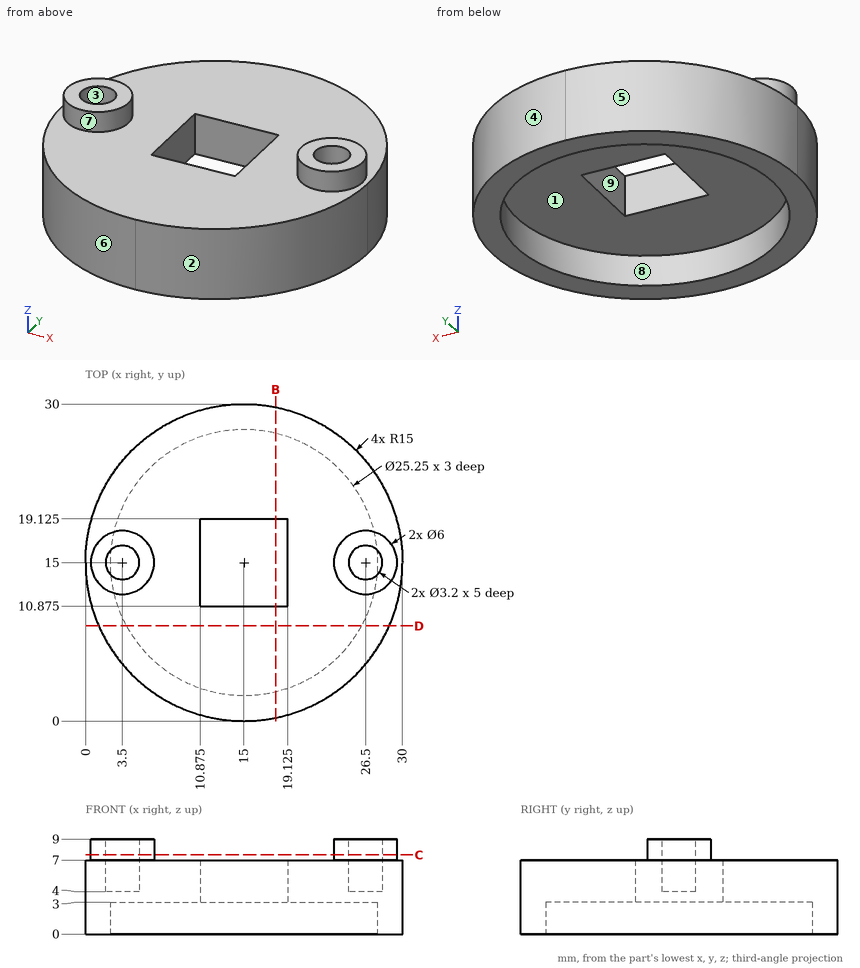
Can you work these out from the drawing? Everything is in mm from the part's minimum corner. A direction names the side the tool comes from. Give positions to 0.01 mm unless a question says otherwise; leave off trailing zeros. Loops run counter-clockwise (first coordinate to the right, second up) from the corner with the lowest first, then second, coordinate; pieces in that order, holes last. Notation, with made-up numbers: (4.25, 77) -> (61.25, 77) arc R7 ccw to (61.25, 82) -> close; hole circle Ø8 at (-27.75, 37.25). An arc over 180 degrees is marked (long way). Write item = value, one per line.
1) Will these pins go through, and if not, where does the flat tip stop? pin 1 (1.5 mm diameter, centred on x = 26, z = 2.5, fed in from -Y); pin 2 (3 mm diameter, centred on x = 3.5, y = 15, fed in from +Z); pin 3 (5 mm diameter, centred on x = 7, y = 8.5, fed in from +Z); pin 4 (5 mm diameter, centred on x = 14, z = 8, fed in from -Y).
Check result:
pin_1 = 4.05
pin_2 = 4
pin_3 = 7
pin_4 = 0
2) For the marked faces 5, 6, 7, 8 and 9, which set-ups out of +Z, -Z, +X, -X, +Y, -Y let a thin tool reach every point of the face, with its end or its side?
Check result:
face_5 = +Z, -Z, -X, +Y
face_6 = +Z, -Z, -X, -Y
face_7 = +Z
face_8 = -Z
face_9 = +Z, -Z
3) Suppose I cut it at C-C on z = 7.5. Write out the boundary of the cut face in (x, y).
Check result:
outline = circle Ø6 at (3.5, 15); circle Ø6 at (26.5, 15); hole circle Ø3.2 at (3.5, 15); hole circle Ø3.2 at (26.5, 15)
4) Thinking about a two-plate mould opening in Y: for the marked faces 1, 2, 3 and 4, which applies, released by +Y, released by -Y, zero draft, split by the parting line, or undercut?
Check result:
face_1 = undercut
face_2 = released by -Y
face_3 = undercut
face_4 = released by +Y
5) Suppose I cut it at B-B on x = 18. Write out the boundary of the cut face in (y, z) (1 decimal).
Check result:
outline = (0.3, 0) -> (2.7, 0) -> (2.7, 3) -> (10.9, 3) -> (10.9, 7) -> (0.3, 7) -> close; (19.1, 3) -> (27.3, 3) -> (27.3, 0) -> (29.7, 0) -> (29.7, 7) -> (19.1, 7) -> close
6) I need wall thicknesses on L1, parallel to Z at x = 19, y = 10; L2, parallel to Y at x = 4, z = 6.75; L3, parallel to X at y = 14, z = 2.75. Which ranges of each line are inside material? Lowest first, please. Write a range as from..to.
Check result:
L1 = 3..7
L2 = 4.8..13.48, 16.52..25.2
L3 = 0.03..2.41, 27.59..29.97
7) Suppose I cut it at D-D on y = 9. Write out the boundary of the cut face in (x, z), then the cut area to 3 significant figures.
Check result:
outline = (1.25, 0) -> (3.89, 0) -> (3.89, 3) -> (26.11, 3) -> (26.11, 0) -> (28.75, 0) -> (28.75, 7) -> (1.25, 7) -> close
area = 126 mm2
